Design review of the part built by this model. Coordinates are the model's own, in mm. A direction names the side the tool comes from. Round coordinates to 2 decimals unless told otherwise and drop trailing zeros. Loops run counter-clockwise (first coordinate to the right, second up) from the corner with the lowest first, then second, coordinate; pieces in that order, holes last. Notation, with made-up numbers: (7, 48) - (37, 48) arc R17 ccw to (37, 70) - close; hole circle Ø5 at (10.25, 20). An arc over 180 degrees is marked (long way). Return JSON: item names as keys, results as strings. Group by question number.
(1) We need section A-A, the plane y = -10.5. Write out the cut boundary in (x, z), and give its area (3 significant figures).
(2) The part is to be moulded in two halves that separate along X. For faces 1 (the cylindrical face through (26.79, -24.82, 9.44)), 2 (the flat face through (-22.669, 22, 4)), 3 (the flat face through (-2, -26, 0)), say which applies: pulls with the +X half, pulls with the -X half, needs draft (parallel to the pull), parting line crosses it, or undercut.
(3) We need section B-B, the plane z = 3. Write out the cut boundary in (x, y), and give its area (3 significant figures).
(4) Clearance check with flat-ended pins moving along their axes: pin 1 (0.8 mm diameter, centred on y = 22, z = 3, fed in from -X); pin 2 (10 mm diameter, centred on x = 14, y = -10.5, fed in from -Z); pin 3 (1 mm diameter, centred on x = 11, y = -8, fed in from +Z). State where each tip first meets the part, or that it passes through.
(5) For faces 4 (the flat face through (-25.562, 25, 9)), 5 (the flat face through (-0.713, 22, 4)), 6 (the flat face through (22, 17.5, 16)), list the 3-axis set-ups (+Z, -Z, +X, -X, +Y, -Y) from which the entire face can be reached by the end or side of a thin tool; tool diameter is ignored.
(6) We need section C-C, the plane x = -8. Write out the cut boundary in (y, z), and give its area (3 significant figures).
(7) Wall thickness on L1, parallel to Y at x = 25.5, z = 9.85; L2, parallel to Y at x = -25.5, z = 9.15; L3, parallel to X at y = 24, z = 15.75: over which ranges is each line inside the solid? List them lowest first. Write a range as [from, to].
(8) We need section D-D, the plane y = 24.5. Write out the cut boundary in (x, z), and give its area (3 significant figures).
from build123d import *

# Parameters (mm, degrees)
SKETCH1_W                      = 57
SKETCH1_H                      = 57
BOSS_EXTRUDE1_DEPTH            = 10.4
SKETCH2_W                      = 7.8
SKETCH2_H                      = 10
BOSS_EXTRUDE3_DEPTH            = 11.7
F_3_5_3_5_DIAMETER_HOLE1_D     = 3.5
F_3_5_3_5_DIAMETER_HOLE1_DEPTH = 10.4
CUT_EXTRUDE1_REACH             = 12.4
SKETCH7_W                      = 21.956188663
SKETCH7_H                      = 2.5
SKETCH7_W_2                    = 42
CUT_EXTRUDE2_DEPTH             = 8.5


with BuildPart() as part:
    # Sketch1 → Boss-Extrude1 (new body)
    with BuildSketch(Plane.XY):
        Rectangle(SKETCH1_W, SKETCH1_H)
    extrude(amount=BOSS_EXTRUDE1_DEPTH)

    # Sketch2 → Boss-Extrude3 (add)
    with BuildSketch(Plane.XY.offset(10.4)):
        with Locations((22.5, 22.5)):
            Rectangle(SKETCH2_W, SKETCH2_H)
    extrude(amount=BOSS_EXTRUDE3_DEPTH)

    # Ø3.5 (3.5) Diameter Hole1
    with Locations(Plane.XY.offset(10.4)):
        with Locations((-25.5, 17.5), (-25.148622044, -10.5), (25.5, -26)):
            Hole(F_3_5_3_5_DIAMETER_HOLE1_D / 2, depth=F_3_5_3_5_DIAMETER_HOLE1_DEPTH)

    # Sketch6 → Cut-Extrude1 (cut, up to next)
    with BuildSketch(Plane.XY.offset(10.4), mode=Mode.PRIVATE) as cut_extrude1_sk1:
        Polygon((-25.562379587, 28.5), (-25.562379587, 21.769543161), (-28.5, 18.222574402), (-28.5, 28.5), align=None)
    cut_extrude1_tool1 = extrude(cut_extrude1_sk1.sketch, amount=-CUT_EXTRUDE1_REACH, mode=Mode.PRIVATE) & part.part
    add(cut_extrude1_tool1.solids().sort_by_distance((-27.133296, 24.186386, 10.4))[0], mode=Mode.SUBTRACT)
    # Sketch6 → Cut-Extrude1 (cut, up to next)
    with BuildSketch(Plane.XY.offset(10.4), mode=Mode.PRIVATE) as cut_extrude1_sk2:
        Polygon((-25.169304276, -15.622117115), (-28.5, -11.638473715), (-28.5, -28.5), (-25.169304276, -28.5), align=None)
    cut_extrude1_tool2 = extrude(cut_extrude1_sk2.sketch, amount=-CUT_EXTRUDE1_REACH, mode=Mode.PRIVATE) & part.part
    add(cut_extrude1_tool2.solids().sort_by_distance((-26.909011, -21.02068, 10.4))[0], mode=Mode.SUBTRACT)

    # Sketch7 → Cut-Extrude2 (cut)
    with BuildSketch(Plane(origin=(0, 0, 0), x_dir=(-1, 0, 0), z_dir=(0, 0, -1))):
        Polygon((-28.5, -28.5), (25.169304276, -28.5), (25.169304276, -15.622117115), (28.5, -11.638473715), (28.5, 18.222574402), (25.562379587, 21.769543161), (25.562379587, 28.5), (-28.5, 28.5), align=None)
        with Locations((11.691209945, 22.5)):
            Rectangle(SKETCH7_W, SKETCH7_H, mode=Mode.SUBTRACT)
        with Locations((1.669304276, -26.25)):
            Rectangle(SKETCH7_W_2, SKETCH7_H, mode=Mode.SUBTRACT)
    extrude(amount=-CUT_EXTRUDE2_DEPTH, mode=Mode.SUBTRACT)


solid = part.part
Solutions:
{
 "1": {"outline": "(-28.5, 8.5) - (-26.9, 8.5) - (-26.9, 10.4) - (-28.5, 10.4) - close; (-23.4, 8.5) - (28.5, 8.5) - (28.5, 10.4) - (-23.4, 10.4) - close", "area": "102 mm^2"},
 "2": {"face 1": "undercut", "face 2": "pulls with the -X half", "face 3": "needs draft"},
 "3": {"outline": "(-22.67, -27.5) - (19.33, -27.5) - (19.33, -25) - (-22.67, -25) - close; (-22.67, 21.25) - (-0.71, 21.25) - (-0.71, 23.75) - (-22.67, 23.75) - close", "area": "160 mm^2"},
 "4": {"pin 1": "x = -22.67", "pin 2": "z = 8.5", "pin 3": "z = 10.4"},
 "5": {"face 4": "+Z, -Z, -X, +Y", "face 5": "-Z, +X, +Y", "face 6": "+Z, +X, -X, -Y"},
 "6": {"outline": "(-28.5, 8.5) - (-27.5, 8.5) - (-27.5, 0) - (-25, 0) - (-25, 8.5) - (21.25, 8.5) - (21.25, 0) - (23.75, 0) - (23.75, 8.5) - (28.5, 8.5) - (28.5, 10.4) - (-28.5, 10.4) - close", "area": "151 mm^2"},
 "7": {"L1": "[-28.5, -27.75], [-24.25, 28.5]", "L2": "[-15.23, -12.21], [-8.79, 15.75], [19.25, 28.5]", "L3": "[18.6, 26.4]"},
 "8": {"outline": "(-25.56, 8.5) - (28.5, 8.5) - (28.5, 10.4) - (26.4, 10.4) - (26.4, 22.1) - (18.6, 22.1) - (18.6, 10.4) - (-25.56, 10.4) - close", "area": "194 mm^2"}
}
